from build123d import *

# Parameters (mm, degrees)
SKETCH1_W           = 150
SKETCH1_H           = 80
BOSS_EXTRUDE1_DEPTH = 50
SKETCH2_W           = 145
SKETCH2_H           = 75
CUT_EXTRUDE1_DEPTH  = 45
SKETCH6_W           = 2.5
SKETCH6_H           = 75
BOSS_EXTRUDE3_DEPTH = 20
SKETCH7_W           = 2.5
SKETCH7_H           = 75
BOSS_EXTRUDE4_DEPTH = 20
SKETCH10_W          = 2.5
SKETCH10_H          = 75
BOSS_EXTRUDE5_DEPTH = 20
SKETCH12_R          = 2.5
CUT_EXTRUDE8_DEPTH  = 10


with BuildPart() as part:
    # Sketch1 → Boss-Extrude1 (new body)
    with BuildSketch(Plane(origin=(0, 0, 0), x_dir=(1, 0, 0), z_dir=(0, 1, 0))):
        Rectangle(SKETCH1_W, SKETCH1_H)
    extrude(amount=BOSS_EXTRUDE1_DEPTH)

    # Sketch2 → Cut-Extrude1 (cut)
    with BuildSketch(Plane(origin=(0, 50, 0), x_dir=(1, 0, 0), z_dir=(0, 1, 0))):
        Rectangle(SKETCH2_W, SKETCH2_H)
    extrude(amount=-CUT_EXTRUDE1_DEPTH, mode=Mode.SUBTRACT)

    # Sketch6 → Boss-Extrude3 (add)
    with BuildSketch(Plane(origin=(0, 5, 0), x_dir=(1, 0, 0), z_dir=(0, 1, 0))):
        Rectangle(SKETCH6_W, SKETCH6_H)
    extrude(amount=BOSS_EXTRUDE3_DEPTH)

    # Sketch7 → Boss-Extrude4 (add)
    with BuildSketch(Plane(origin=(0, 5, 0), x_dir=(1, 0, 0), z_dir=(0, 1, 0))):
        with Locations((-39.404677113, 0)):
            Rectangle(SKETCH7_W, SKETCH7_H)
    extrude(amount=BOSS_EXTRUDE4_DEPTH)

    # Sketch10 → Boss-Extrude5 (add)
    with BuildSketch(Plane(origin=(0, 5, 0), x_dir=(1, 0, 0), z_dir=(0, 1, 0))):
        with Locations((36.606323204, 0)):
            Rectangle(SKETCH10_W, SKETCH10_H)
    extrude(amount=BOSS_EXTRUDE5_DEPTH)

    # Sketch12 → Cut-Extrude8 (cut)
    with BuildSketch(Plane(origin=(75, 0, 0), x_dir=(0, 0, -1), z_dir=(1, 0, 0))):
        with Locations((0, 30)):
            Circle(SKETCH12_R)
    extrude(amount=-CUT_EXTRUDE8_DEPTH, mode=Mode.SUBTRACT)


solid = part.part
Geometry check sheet. Reference: the model listing, model coordinates, mm. A direction names the side the tool comes from. Give positions to 0.01 mm unless a question says otherwise; leave off trailing zeros. Loops run counter-clockwise (first coordinate to the right, second up) from the corner with the lowest first, then second, coordinate; pieces in that order, holes last.
(1) Section check C-C on y = 39.5. Record the cut outline in (x, z).
From the geometry:
outline: (-75, -40) - (75, -40) - (75, 40) - (-75, 40) - close; hole (-72.5, -37.5) - (72.5, -37.5) - (72.5, 37.5) - (-72.5, 37.5) - close
(2) Thickness scan on L1, parallel to X at y = 18, z = -22.5; L2, parallel to Z at x = 12, y = 24; L3, parallel to X at y = 39, z = 25. Record the ranges inside material, lowest first.
From the geometry:
L1: x = -75 to -72.5, -40.65 to -38.15, -1.25 to 1.25, 35.36 to 37.86, 72.5 to 75
L2: z = -40 to -37.5, 37.5 to 40
L3: x = -75 to -72.5, 72.5 to 75
(3) Release check for a two-part mould opening along Z. For faces 1 (the flat face through (-38.155, 15, 1)), 2 (the flat face through (-1, 0, -1)), 3 (the flat face through (18, 5, -1)) record: released by +Z, released by -Z, zero draft, split by the parting line, or undercut.
From the geometry:
face 1: undercut
face 2: zero draft
face 3: undercut
(4) Section check B-B on y = 30. Record the cut outline in (x, z), then the cut area to 3 significant figures.
From the geometry:
outline: (-75, -40) - (75, -40) - (75, -2.5) - (72.5, -2.5) - (72.5, -37.5) - (-72.5, -37.5) - (-72.5, 37.5) - (72.5, 37.5) - (72.5, 2.5) - (75, 2.5) - (75, 40) - (-75, 40) - close
area: 1,110 mm2
(5) Section check D-D on y = 15.5. Record the cut outline in (x, z).
From the geometry:
outline: (-75, -40) - (75, -40) - (75, 40) - (-75, 40) - close; hole (-72.5, -37.5) - (-40.65, -37.5) - (-40.65, 37.5) - (-72.5, 37.5) - close; hole (-38.15, -37.5) - (-1.25, -37.5) - (-1.25, 37.5) - (-38.15, 37.5) - close; hole (1.25, -37.5) - (35.36, -37.5) - (35.36, 37.5) - (1.25, 37.5) - close; hole (37.86, -37.5) - (72.5, -37.5) - (72.5, 37.5) - (37.86, 37.5) - close
(6) Section check A-A on z = 0. Record the cut outline in (x, y), then the cut area to 3 significant figures.
From the geometry:
outline: (-75, 0) - (75, 0) - (75, 27.5) - (72.5, 27.5) - (72.5, 5) - (37.86, 5) - (37.86, 25) - (35.36, 25) - (35.36, 5) - (1.25, 5) - (1.25, 25) - (-1.25, 25) - (-1.25, 5) - (-38.15, 5) - (-38.15, 25) - (-40.65, 25) - (-40.65, 5) - (-72.5, 5) - (-72.5, 50) - (-75, 50) - close; (72.5, 32.5) - (75, 32.5) - (75, 50) - (72.5, 50) - close
area: 1,110 mm2
(7) Set-up check for faces 4 (the flat face through (-40.655, 15, 1)), 5 (the cylindrical face through (73.77, 32.11, -1.34)), 6 (the flat face through (-75, 25, 1)): record each of +Z, -Z, +X, -X, +Y, -Y from which the full face is reachable in a straight line by a thin tool's end or side.
From the geometry:
face 4: +Y
face 5: +X
face 6: +Z, -Z, -X, +Y, -Y
(8) Depth check by flat-ended pin: pin 1 Ø1.2 at (x, z) = (-39.5, 3.5) entering from +Y; pin 2 Ø9.5 at (x, z) = (-64.5, -8.5) entering from +Y. Enter the tip coordinate at first touch or a pass-through.
From the geometry:
pin 1: stops at y = 25
pin 2: stops at y = 5
